Input: part model. Units: mm. Frame: model coordinates. Coordinates: 2 decimals unless noted, no trailing zeros. Loops run counter-clockwise (first coordinate to the right, second up) from the corner with the lowest first, then second, coordinate; pieces in that order, holes last.
Item 1: Pull-direction query (Y, two-part tool) for faces 1 (the cylindrical face through (223.163, -34.393, 3.131)), 2 (the flat face through (205.7, 50.22, 3.13)), 3 (the flat face through (4, 17, 0)); classes: released by +Y, released by -Y, zero draft, split by the parting line, or undercut.
Item 2: Section B-B on x = 197. Return loops of the section in (y, z), and give its area (3 significant figures).
Item 3: Ray query, line 1 along X through (y, z) = (28.5, 4); line 2 along X through (y, z) = (1.5, 2.5); line 3 along Y through (x, z) = (-30.5, 2.25). Return the intervals inside material, ascending.
Item 4: Section A-A on z = 1.5. Give the number of separate pieces and of enclosed holes in the cut face, and give its area (3 significant figures).
Item 5: Contact query for a flat-ended pin moving along its axis: P1, Ø2, axis at x = 220.06, y = -31.75, coming from the +Z side. Output: stop coordinate, or through.
```python
from build123d import *

# Parameters (mm, degrees)
SKETCH1_R           = 2.35
SKETCH1_R_2         = 1.85000011
SKETCH1_R_3         = 1.85
BOSS_EXTRUDE1_DEPTH = 6.35


with BuildPart() as part:
    # Sketch1 → Boss-Extrude1 (new body)
    with BuildSketch(Plane.XY):
        with BuildLine():
            Line((-149.618797812, -37.447756374), (-217.287383527, -37.447756374))
            ThreePointArc((-217.287383527, -37.447756374), (-221.777511587, -35.587884435), (-223.637383527, -31.097756374))
            Line((-223.637383527, -31.097756374), (-223.637383527, 33.765977424))
            ThreePointArc((-223.637383527, 33.765977424), (-222.309818874, 38.787300541), (-218.674059542, 42.49639313))
            Line((-218.674059542, 42.49639313), (-190.732762109, 59.128117792))
            ThreePointArc((-190.732762109, 59.128117792), (-171.969166759, 67.120649159), (-151.757691995, 69.85))
            Line((-151.757691995, 69.85), (151.757691995, 69.85))
            ThreePointArc((151.757691995, 69.85), (171.969166759, 67.120649159), (190.732762109, 59.128117792))
            Line((190.732762109, 59.128117792), (221.096676015, 41.054359515))
            ThreePointArc((221.096676015, 41.054359515), (224.732435347, 37.345266926), (226.06, 32.323943809))
            Line((226.06, 32.323943809), (226.06, -27.287756374))
            ThreePointArc((226.06, -27.287756374), (223.084204897, -34.471961271), (215.9, -37.447756374))
            Line((215.9, -37.447756374), (-149.618797812, -37.447756374))
        make_face()
        with Locations((-172.72, 0)):
            Circle(SKETCH1_R, mode=Mode.SUBTRACT)
        with Locations((-57.57418, 0)):
            Circle(SKETCH1_R, mode=Mode.SUBTRACT)
        with Locations((57.5724782, 0)):
            Circle(SKETCH1_R, mode=Mode.SUBTRACT)
        with Locations((172.72, 0)):
            Circle(SKETCH1_R, mode=Mode.SUBTRACT)
        with Locations((220.058830169, -31.752755237)):
            Circle(SKETCH1_R_2, mode=Mode.SUBTRACT)
        with Locations((115.1462391, 27.951065379)):
            Circle(SKETCH1_R, mode=Mode.SUBTRACT)
        with Locations((-220.058830169, -31.752755237)):
            Circle(SKETCH1_R_2, mode=Mode.SUBTRACT)
        with Locations((-32.17418, 60.325)):
            Circle(SKETCH1_R_3, mode=Mode.SUBTRACT)
        with Locations((-152.82418, 60.325)):
            Circle(SKETCH1_R_3, mode=Mode.SUBTRACT)
        with Locations((152.82418, 60.325)):
            Circle(SKETCH1_R_3, mode=Mode.SUBTRACT)
        with Locations((32.17418, 60.325)):
            Circle(SKETCH1_R_3, mode=Mode.SUBTRACT)
        with Locations((115.1453882, -9.897181959)):
            Circle(SKETCH1_R_3, mode=Mode.SUBTRACT)
        with Locations((-115.14709, -9.897181959)):
            Circle(SKETCH1_R_3, mode=Mode.SUBTRACT)
        with Locations((-0.00127, -9.897181959)):
            Circle(SKETCH1_R_3, mode=Mode.SUBTRACT)
        with Locations((220.058830169, 33.81345012)):
            Circle(SKETCH1_R_3, mode=Mode.SUBTRACT)
        with Locations((-220.058830169, 33.81345012)):
            Circle(SKETCH1_R_3, mode=Mode.SUBTRACT)
    extrude(amount=BOSS_EXTRUDE1_DEPTH)


solid = part.part
```
Results found:
1. face 1: released by -Y
1. face 2: released by +Y
1. face 3: zero draft
2. outline: (-37.45, 0) - (55.4, 0) - (55.4, 6.35) - (-37.45, 6.35) - close
2. area: 590 mm2
3. line 1: x = -223.64 to 112.86, 117.43 to 226.06
3. line 2: x = -223.64 to -174.53, -170.91 to -59.38, -55.77 to 55.76, 59.38 to 170.91, 174.53 to 226.06
3. line 3: y = -37.45 to 59.54, 61.11 to 69.85
4. separate pieces: 1
4. enclosed holes: 16
4. area: 46,300 mm2
5. P1: passes through
